Geometry: final body of the model. Coordinates: model frame, mm. Round coordinates to 2 decimals unless told otherwise and drop trailing zeros. Loops run counter-clockwise (first coordinate to the right, second up) from the corner with the lowest first, then second, coordinate; pieces in that order, holes last. Notation, with made-up numbers: (68.5, 80) -> (88.5, 80) arc R9 ccw to (88.5, 86) -> close; hole circle Ø4 at (60.5, 5). An arc over 180 degrees is marked (long way). Answer in a Markdown table with one row per item.
```python
from build123d import *

# Parameters (mm, degrees)
SKETCH1_R           = 75
BOSS_EXTRUDE1_DEPTH = 20
CUT_EXTRUDE1_REACH  = 109.935
SKETCH2_R           = 2.5


with BuildPart() as part:
    # Sketch1 → Boss-Extrude1 (new body)
    with BuildSketch(Plane(origin=(0, 0, 0), x_dir=(1, 0, 0), z_dir=(0, 1, 0))):
        with Locations(Location((0, 0, 0), (0, 0, 270))):
            Circle(SKETCH1_R)
    extrude(amount=BOSS_EXTRUDE1_DEPTH)

    # Sketch2 → Cut-Extrude1 (cut, up to next)
    with BuildSketch(Plane(origin=(0, 20, 0), x_dir=(1, 0, 0), z_dir=(0, 1, 0)), mode=Mode.PRIVATE) as cut_extrude1_sk1:
        with Locations(Location((0, 41.5, 0), (0, 0, 270))):
            Circle(SKETCH2_R)
    cut_extrude1_tool1 = extrude(cut_extrude1_sk1.sketch, amount=-CUT_EXTRUDE1_REACH, mode=Mode.PRIVATE) & part.part
    # Sketch2 → Cut-Extrude1 (cut, up to next)
    with BuildSketch(Plane(origin=(0, 20, 0), x_dir=(1, 0, 0), z_dir=(0, 1, 0)), mode=Mode.PRIVATE) as cut_extrude1_sk2:
        with Locations(Location((41.5, 0, 0), (0, 0, 270))):
            Circle(SKETCH2_R)
    cut_extrude1_tool2 = extrude(cut_extrude1_sk2.sketch, amount=-CUT_EXTRUDE1_REACH, mode=Mode.PRIVATE) & part.part
    # Sketch2 → Cut-Extrude1 (cut, up to next)
    with BuildSketch(Plane(origin=(0, 20, 0), x_dir=(1, 0, 0), z_dir=(0, 1, 0)), mode=Mode.PRIVATE) as cut_extrude1_sk3:
        with Locations(Location((0, -41.5, 0), (0, 0, 270))):
            Circle(SKETCH2_R)
    cut_extrude1_tool3 = extrude(cut_extrude1_sk3.sketch, amount=-CUT_EXTRUDE1_REACH, mode=Mode.PRIVATE) & part.part
    # Sketch2 → Cut-Extrude1 (cut, up to next)
    with BuildSketch(Plane(origin=(0, 20, 0), x_dir=(1, 0, 0), z_dir=(0, 1, 0)), mode=Mode.PRIVATE) as cut_extrude1_sk4:
        with Locations(Location((-41.5, 0, 0), (0, 0, 270))):
            Circle(SKETCH2_R)
    cut_extrude1_tool4 = extrude(cut_extrude1_sk4.sketch, amount=-CUT_EXTRUDE1_REACH, mode=Mode.PRIVATE) & part.part
    add(cut_extrude1_tool1.solids().sort_by_distance((0, 20, -41.5))[0], mode=Mode.SUBTRACT)
    add(cut_extrude1_tool2.solids().sort_by_distance((41.5, 20, 0))[0], mode=Mode.SUBTRACT)
    add(cut_extrude1_tool3.solids().sort_by_distance((0, 20, 41.5))[0], mode=Mode.SUBTRACT)
    add(cut_extrude1_tool4.solids().sort_by_distance((-41.5, 20, 0))[0], mode=Mode.SUBTRACT)


solid = part.part
```
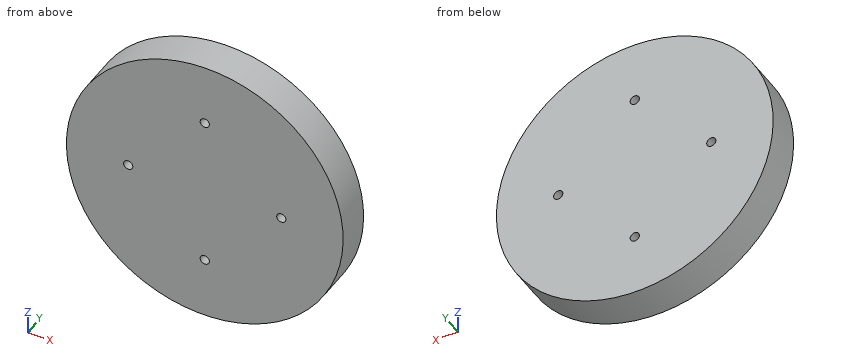
Item 1: Section query D-D, the plane x = -41.5. Output: boundary loops of the cut face in (y, z).
Ans:
| item | result |
|---|---|
| outline | (0, -62.47) -> (20, -62.47) -> (20, -2.5) -> (0, -2.5) -> close; (0, 2.5) -> (20, 2.5) -> (20, 62.47) -> (0, 62.47) -> close |
Item 2: First-contact query: P1, Ø6, axis at x = -3.5, y = 15, coming from the +Z side; P2, Ø4, axis at y = 4, z = 55.5, coming from the +X side; P3, Ø10, axis at y = 3, z = 19.5, coming from the +X side (3 decimals); P4, Ø4.5, axis at x = 0, z = -41.5, coming from the +Y side. Flat tips, straight axial feed; report the tip coordinate or a pass-through.
Ans:
| item | result |
|---|---|
| P1 | z = 75 |
| P2 | x = 52.56 |
| P3 | x = 73.585 |
| P4 | through |
Item 3: Ray query, L1, parallel to X at y = 12.25, z = 0; L2, parallel to X at y = 5.75, z = 41.5; L3, parallel to Z at x = -41, y = 19. Return the intervals inside material, ascending.
Ans:
| item | result |
|---|---|
| L1 | -75 to -44, -39 to 39, 44 to 75 |
| L2 | -62.47 to -2.5, 2.5 to 62.47 |
| L3 | -62.8 to -2.45, 2.45 to 62.8 |
Item 4: Section query C-C, the plane y = 3.5. Output: boundary loops of the cut face in (x, z).
Ans:
| item | result |
|---|---|
| outline | circle Ø150 at (0, 0); hole circle Ø5 at (-41.5, 0); hole circle Ø5 at (0, -41.5); hole circle Ø5 at (0, 41.5); hole circle Ø5 at (41.5, 0) |
Item 5: Section query B-B, the plane z = -41.5. Output: boundary loops of the cut face in (x, y).
Ans:
| item | result |
|---|---|
| outline | (-62.47, 0) -> (-2.5, 0) -> (-2.5, 20) -> (-62.47, 20) -> close; (2.5, 0) -> (62.47, 0) -> (62.47, 20) -> (2.5, 20) -> close |
Item 6: Section query A-A, the plane x = 0. Output: boundary loops of the cut face in (y, z).
Ans:
| item | result |
|---|---|
| outline | (0, -75) -> (20, -75) -> (20, -44) -> (0, -44) -> close; (0, -39) -> (20, -39) -> (20, 39) -> (0, 39) -> close; (0, 44) -> (20, 44) -> (20, 75) -> (0, 75) -> close |
